For this review, take the finished solid that the model builds, in its own axes (mm). Round coordinates to 2 decimals unless told otherwise and drop trailing zeros. Write each loop counter-clockwise with the first axis right and the second up, starting at its lowest first coordinate (ties: lowest second). Pieces come first, ordered by that corner, then holes. Notation, with made-up numbers: (69.5, -5) - (89.5, -5) arc R28 ccw to (89.5, 13) - close; hole circle Ø7 at (86.5, 83). An arc over 180 degrees is marked (long way). One line per item, written item: value. Start each with the question number.
Q1. Clearance check with flat-ended pins moving along their axes: pin 1 Ø0.9 at (y, z) = (106, 2) entering from -X; pin 2 Ø1.4 at (y, z) = (105.5, 2) entering from +X; pin 3 Ø0.9 at (x, z) = (6, 1.5) entering from +Y. State where each tip first meets the part, or that it passes through.
Q2. Add section B-B on y = 2. Write out the cut boundary in (x, z).
Q3. For probe 1 along X at (y, z) = (-31, 2.6); probe 2 along Y at (x, z) = (-16, 0.4); probe 3 along Y at (x, z) = (129.5, 2.65), list the stretches that pass through material, from the lowest coordinate up.
Q4. Add section A-A on x = 72.5. Write out the cut boundary in (y, z).
Q5. Mouldability with a two-part tool opening along Y and no side actions: class faces 1 (the face through (152.907, -64.568, 1.479)), 2 (the face through (-15, 17, 3)), 3 (the face through (102.105, 44.498, 1.521)) as +Y half, -Y half, draft (parallel to the pull), parting line (faces both ways), or undercut.
```python
from build123d import *

# Parameters (mm, degrees)
BOSS_EXTRUDE1_DEPTH = 3
CUT_EXTRUDE2_DEPTH  = 3
LPATTERN2_COUNT     = 6
LPATTERN2_PITCH     = 25
CUT_EXTRUDE3_DEPTH  = 3
LPATTERN3_COUNT     = 6
LPATTERN3_PITCH     = 25
CAVITY4_START       = 94.102573719
CAVITY4_DEPTH       = 3
SKETCH4_W           = 10
SKETCH4_H           = 3
SKETCH4_W_2         = 15.058056796
SKETCH4_H_2         = 3.003228899
CUT_EXTRUDE5_DEPTH  = 10


# Read off the part's stored shape, not the designer's step: Cavity4
with BuildPart() as part:
    # Sketch1 → Boss-Extrude1 (new body)
    with BuildSketch(Plane.XY):
        Polygon((-182.169109633, -75.86705578), (157.830890367, -75.86705578), (77.830890367, 107.708711956), (-102.169109633, 107.708711956), align=None)
    extrude(amount=BOSS_EXTRUDE1_DEPTH)

    # Sketch2 → Cut-Extrude2 (cut)
    with BuildSketch(Plane.XY.offset(3)):
        Polygon((-172.181594028, -52.948732717), (-169.400999714, -54.074918874), (-164.054462817, -40.06012158), (-166.030438991, -38.833695112), align=None)
    cut_extrude2 = extrude(amount=-CUT_EXTRUDE2_DEPTH, mode=Mode.SUBTRACT)

    # LPattern2: Cut-Extrude2 ×6
    with Locations(*[Vector(0.3995006242197252, 0.916732922528721, 0) * (i * LPATTERN2_PITCH) for i in range(1, LPATTERN2_COUNT)]):
        add(cut_extrude2, mode=Mode.SUBTRACT)

    # Sketch3 → Cut-Extrude3 (cut)
    with BuildSketch(Plane.XY.offset(3)):
        Polygon((147.843374761, -52.948732717), (141.850865398, -39.197738879), (139.10066663, -40.396240752), (145.093175994, -54.14723459), align=None)
    cut_extrude3 = extrude(amount=-CUT_EXTRUDE3_DEPTH, mode=Mode.SUBTRACT)

    # LPattern3: Cut-Extrude3 ×6
    with Locations(*[Vector(-0.3995006242197251, 0.9167329225287211, 0) * (i * LPATTERN3_PITCH) for i in range(1, LPATTERN3_COUNT)]):
        add(cut_extrude3, mode=Mode.SUBTRACT)

    # Cavity4 outline → Cavity4 (cut)
    with BuildSketch(Plane(origin=(0, 0, 0), x_dir=(0.9999532933915303, -0.008562000513036364, -0.004483657284732639), z_dir=(0.009664938459823271, 0.8858411925353571, 0.46388788577856205)).offset(CAVITY4_START)):
        Polygon((-103.131187753, 49.679443772), (-88.131836909, 49.53989356), (-88.127862283, 49.967100463), (-88.118252444, 51), (-103.118901627, 51), (-103.12893984, 49.921057402), align=None)
        Polygon((-63.117170469, 51), (-73.117603258, 51), (-73.127213098, 49.967100463), (-73.132486065, 49.400343349), (-63.132918836, 49.307309875), (-63.126780309, 49.967100463), align=None)
        Polygon((-38.116088496, 51), (-48.116521286, 51), (-48.126131125, 49.967100463), (-48.133567992, 49.167759664), (-38.134000762, 49.07472619), (-38.125698335, 49.967100463), align=None)
        Polygon((-13.115006523, 51), (-23.115439311, 51), (-23.125049151, 49.967100463), (-23.134649919, 48.935175979), (-13.135082689, 48.842142504), (-13.124616362, 49.967100463), align=None)
        Polygon((76.879278743, 49.967100463), (76.888888582, 51), (51.887806609, 51), (51.87819677, 49.967100463), (51.862104301, 48.237424923), (76.861022374, 48.004841237), align=None)
        Polygon((11.886075451, 51), (1.885642662, 51), (1.876032823, 49.967100463), (1.864268155, 48.702592293), (11.863835384, 48.609558819), (11.876465612, 49.967100463), align=None)
        Polygon((36.877547586, 49.967100463), (36.887157425, 51), (26.886724635, 51), (26.877114796, 49.967100463), (26.863186228, 48.470008608), (36.862753457, 48.376975134), align=None)
    extrude(amount=CAVITY4_DEPTH, mode=Mode.SUBTRACT)

    # Sketch4 → Cut-Extrude5 (cut)
    with BuildSketch(Plane(origin=(0, 0, 0), x_dir=(-1, 0, 0), z_dir=(0, 0, -1))):
        Polygon((-77.830853836, 107.708711956), (-77.830853836, 104.708711956), (-52.830853836, 104.708711956), (-52.795526537, 107.708711956), align=None)
        with Locations((-32.830890367, 106.241816524)):
            Rectangle(SKETCH4_W, SKETCH4_H)
        with Locations((-7.830890367, 106.241816524)):
            Rectangle(SKETCH4_W, SKETCH4_H)
        with Locations((17.169109633, 106.241816524)):
            Rectangle(SKETCH4_W, SKETCH4_H)
        with Locations((42.169109633, 106.241816524)):
            Rectangle(SKETCH4_W, SKETCH4_H)
        with Locations((67.169109633, 106.241816524)):
            Rectangle(SKETCH4_W, SKETCH4_H)
        with Locations((94.698138031, 106.243430974)):
            Rectangle(SKETCH4_W_2, SKETCH4_H_2)
    extrude(amount=-CUT_EXTRUDE5_DEPTH, mode=Mode.SUBTRACT)


solid = part.part
```
Result set:
1. pin 1: stops at x = -103.11
1. pin 2: stops at x = 79.1
1. pin 3: stops at y = 104.74
2. outline: (-145.52, 0) - (120.62, 0) - (120.62, 3) - (-145.52, 3) - close
3. probe 1: x = -162.62 to -159.8, -159.35 to 135.01, 135.63 to 138.28
3. probe 2: y = -75.87 to 104.74
3. probe 3: y = -75.87 to -18.37, -17.31 to -10.86
4. outline: (-75.87, 0) - (104.71, 0) - (104.71, 3) - (-75.87, 3) - close
5. face 1: +Y half
5. face 2: draft
5. face 3: undercut
